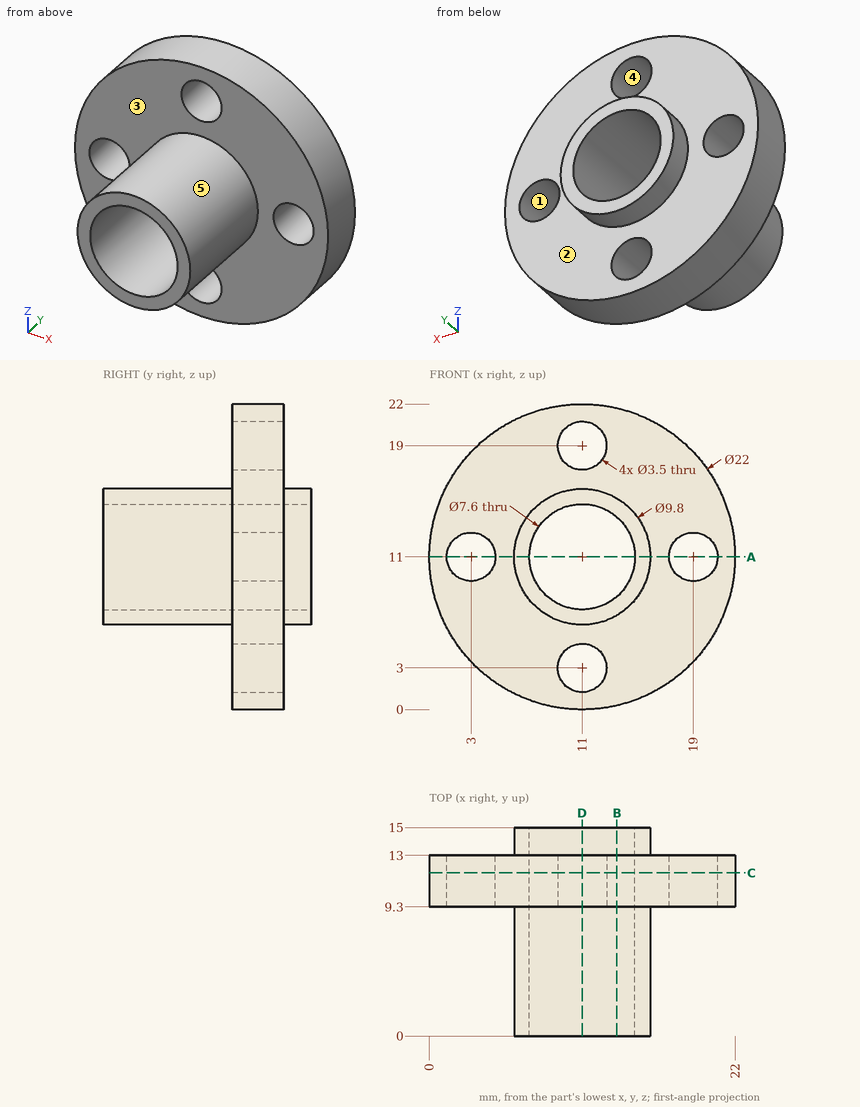
The figure shows three views and two pictorial views of one solid part (mm, origin at its lowest corner). Answer the questions. A direction names the side the tool comes from. Round coordinates to 2 decimals unless told otherwise and drop trailing zeros. Loops run counter-clockwise (first coordinate to the right, second up) from the corner with the lowest first, then second, coordinate; pieces in that order, holes last. Notation, with made-up numbers: M 21.25,-2 L 80.25,-2 A18 cw 80.25,17 Z; hole C 7,21 d1. An arc over 180 degrees is marked long. Write each question's results on one line, items separated by ' | '. Start each with the question number.
1) Determine the mould class of the marked faces 3, 4 and 5 for opening direction Z: pulls with the +Z half, pulls with the -Z half, needs draft (parallel to the pull), parting line crosses it, or undercut.
2) Find section A-A on z = 11. Write down the section's boundary in (x, y).
3) Each of these flat-tipped pins is pushed along its axis until it touches: pin 1 (5 mm diameter, centred on x = 11, y = 4.5, fed in from +Z); pin 2 (4 mm diameter, centred on x = 19, z = 11, fed in from +Y); pin 3 (2 mm diameter, centred on x = 5, y = 10, fed in from -Z); pin 4 (4.5 mm diameter, centred on x = 11, z = 11, fed in from +Y). Where does it stop, or does it pass through?
4) Find section D-D on x = 11. Write down the section's boundary in (y, z), plus the area to 3 significant figures.
5) Find section B-B on x = 13.5. Write down the section's boundary in (y, z), plus the area to 3 significant figures.
6) Straight lines are drawn through the part: probe 1 along X at (y, z) = (11.05, 11); probe 2 along Y at (x, z) = (16.5, 15.5). For each, find the intervals that lie inside material, in ascending order.
7) Which of the six approach directions +Z, -Z, +X, -X, +Y, -Y give full straight-line access (tool end or side, diameter ignored) to the marked faces 1 and 2?
8) Find section C-C on y = 11.75. Write down the section's boundary in (x, z), plus the area to 3 significant figures.
Final values:
1) face 3: needs draft | face 4: undercut | face 5: parting line crosses it
2) outline: M 0,9.3 L 1.25,9.3 L 1.25,13 L 0,13 Z; M 4.75,9.3 L 6.1,9.3 L 6.1,0 L 7.2,0 L 7.2,15 L 6.1,15 L 6.1,13 L 4.75,13 Z; M 14.8,0 L 15.9,0 L 15.9,9.3 L 17.25,9.3 L 17.25,13 L 15.9,13 L 15.9,15 L 14.8,15 Z; M 20.75,9.3 L 22,9.3 L 22,13 L 20.75,13 Z
3) pin 1: z = 15.9 | pin 2: y = 13 | pin 3: z = 1.2 | pin 4: through
4) outline: M 0,6.1 L 9.3,6.1 L 9.3,4.75 L 13,4.75 L 13,6.1 L 15,6.1 L 15,7.2 L 0,7.2 Z; M 0,14.8 L 15,14.8 L 15,15.9 L 13,15.9 L 13,17.25 L 9.3,17.25 L 9.3,15.9 L 0,15.9 Z; M 9.3,0 L 13,0 L 13,1.25 L 9.3,1.25 Z; M 9.3,20.75 L 13,20.75 L 13,22 L 9.3,22 Z | area: 52.2 mm²
5) outline: M 0,6.79 L 9.3,6.79 L 9.3,0.29 L 13,0.29 L 13,6.79 L 15,6.79 L 15,8.14 L 0,8.14 Z; M 0,13.86 L 15,13.86 L 15,15.21 L 13,15.21 L 13,21.71 L 9.3,21.71 L 9.3,15.21 L 0,15.21 Z | area: 88.7 mm²
6) probe 1: 0 to 1.25, 4.75 to 7.2, 14.8 to 17.25, 20.75 to 22 | probe 2: 9.3 to 13
7) face 1: +Y, -Y | face 2: +Y
8) outline: C 11,11 d22; hole C 3,11 d3.5; hole C 11,11 d7.6; hole C 11,3 d3.5; hole C 11,19 d3.5; hole C 19,11 d3.5 | area: 296 mm²
